Could you check a few things on this model? Use its own coordinates, in mm. Give positions to 0.01 mm unless a question says otherwise; leave off trailing zeros. Loops run counter-clockwise (first coordinate to the right, second up) from the corner with the lowest first, then second, coordinate; pieces in that order, holes last. Notation, with made-up numbers: (24.5, 21) - (72.5, 21) arc R31 ccw to (72.5, 45) - close; hole circle Ø1 at (14.5, 52.25). An arc over 180 degrees is marked (long way). Use CSV: the item, a comma, the result in double quotes.
from build123d import *

# Parameters (mm, degrees)
ESBO_O1_W                         = 130
ESBO_O1_H                         = 55.25
RESSALTO_EXTRUS_O1_DEPTH          = 2.5
ESBO_O2_W                         = 130
ESBO_O2_H                         = 55.25
ESBO_O2_W_2                       = 125
ESBO_O2_H_2                       = 50.25
CORTE_EXTRUS_O1_DEPTH             = 1.25
FUROS_GUIA_COM_3_0MM2_D           = 3
FUROS_GUIA_COM_3_0MM2_CSINK_D     = 3.05
FUROS_GUIA_COM_3_0MM2_CSINK_ANGLE = 90
CUT_EXTRUDE1_DEPTH                = 10
FILETE1_R                         = 2
FURO_COM_FOLGA_DE_M21_D           = 2.4
PADR_O_LINEAR1_COUNT              = 3
PADR_O_LINEAR1_PITCH              = 8
ESPELHAR1_COPY_1_D                = 2.4
ESPELHAR1_COPY_2_D                = 2.4
ESPELHAR2_COPY_1_D                = 2.4
ESPELHAR2_COPY_2_D                = 2.4
ESPELHAR2_COPY_3_D                = 2.4
ESPELHAR2_COPY_4_D                = 2.4
ESPELHAR2_COPY_5_D                = 2.4
FILETE1_OF_ESPELHAR2_R            = 2


with BuildPart() as part:
    # Esboço1 → Ressalto-extrusão1 (new body)
    with BuildSketch(Plane.XY):
        with Locations((1.708397535, 5.726309707)):
            Rectangle(ESBO_O1_W, ESBO_O1_H)
    extrude(amount=RESSALTO_EXTRUS_O1_DEPTH)

    # Esboço2 → Corte-extrusão1 (cut)
    with BuildSketch(Plane.XY.offset(2.5)):
        with Locations((1.708397535, 5.726309707)):
            Rectangle(ESBO_O2_W, ESBO_O2_H)
        with Locations((1.708397535, 5.726309707)):
            Rectangle(ESBO_O2_W_2, ESBO_O2_H_2, mode=Mode.SUBTRACT)
    extrude(amount=-CORTE_EXTRUS_O1_DEPTH, mode=Mode.SUBTRACT)

    # Furos-guia com Ø3.0mm2 (through all)
    with Locations(Plane.XY.offset(2.5)):
        with Locations((-48.791602465, 22.551309707), (-48.791602465, -11.098690293), (52.208397535, -11.098690293), (52.208397535, 22.551309707)):
            CounterSinkHole(FUROS_GUIA_COM_3_0MM2_D / 2, FUROS_GUIA_COM_3_0MM2_CSINK_D / 2, counter_sink_angle=FUROS_GUIA_COM_3_0MM2_CSINK_ANGLE)

    # Sketch1 → Cut-Extrude1 (cut)
    with BuildSketch(Plane.XY.offset(2.5)):
        with BuildLine():
            Line((-39.291602465, -4.773695916), (-15.791602465, -4.773695916))
            Line((-15.791602465, -4.773695916), (-15.791602465, 16.226304084))
            Line((-15.791602465, 16.226304084), (-39.291602465, 16.226304084))
            ThreePointArc((-39.291602465, 16.226304084), (-43.887668713, 13.19109981), (-49.291602465, 12.126304084))
            ThreePointArc((-49.291602465, 12.126304084), (-55.691602465, 5.726304084), (-49.291602465, -0.673695916))
            ThreePointArc((-49.291602465, -0.673695916), (-43.887668713, -1.738491642), (-39.291602465, -4.773695916))
        make_face()
    cut_extrude1 = extrude(amount=-CUT_EXTRUDE1_DEPTH, mode=Mode.SUBTRACT)

    # Filete1
    filete1_edges = [part.edges().sort_by_distance(p)[0] for p in [
        (-39.291602465, -4.773695916, 1.25),
        (-39.291602465, 16.226304084, 1.25),
        (-15.791602465, 16.226304084, 1.25),
        (-15.791602465, -4.773695916, 1.25),
    ]]
    fillet(filete1_edges, radius=FILETE1_R)

    # Furo com folga de M21 (through all)
    with Locations(Plane.XY.offset(2.5)):
        with Locations((37.958397535, -7.773690293)):
            furo_com_folga_de_m21 = Hole(FURO_COM_FOLGA_DE_M21_D / 2)

    # Padrão linear1: Furo com folga de M21 ×3
    with Locations(*[(-i * PADR_O_LINEAR1_PITCH, 0, 0) for i in range(1, PADR_O_LINEAR1_COUNT)]):
        add(furo_com_folga_de_m21, mode=Mode.SUBTRACT)

    # Espelhar1: Furo com folga de M21 across plane
    add(furo_com_folga_de_m21.mirror(Plane(origin=(0, 5.726309707, 0), x_dir=(0, 0, 1), z_dir=(0, -1, 0))), mode=Mode.SUBTRACT)

    # Espelhar1 copy 1 (through all)
    with Locations(Plane(origin=(-8, 11.452619414, 2.5), x_dir=(1, 0, 0), z_dir=(0, 0, 1))):
        with Locations((37.958397535, 7.773690293)):
            Hole(ESPELHAR1_COPY_1_D / 2)

    # Espelhar1 copy 2 (through all)
    with Locations(Plane(origin=(-16, 11.452619414, 2.5), x_dir=(1, 0, 0), z_dir=(0, 0, 1))):
        with Locations((37.958397535, 7.773690293)):
            Hole(ESPELHAR1_COPY_2_D / 2)

    # Espelhar2: Cut-Extrude1, Furo com folga de M21 across plane
    add(cut_extrude1.mirror(Plane(origin=(1.708397535, 0, 0), x_dir=(0, 0, 1), z_dir=(1, 0, 0))), mode=Mode.SUBTRACT)
    add(furo_com_folga_de_m21.mirror(Plane(origin=(1.708397535, 0, 0), x_dir=(0, 0, 1), z_dir=(1, 0, 0))), mode=Mode.SUBTRACT)

    # Espelhar2 copy 1 (through all)
    with Locations(Plane(origin=(11.416795069, 0, 2.5), x_dir=(-1, 0, 0), z_dir=(0, 0, 1))):
        with Locations((37.958397535, 7.773690293)):
            Hole(ESPELHAR2_COPY_1_D / 2)

    # Espelhar2 copy 2 (through all)
    with Locations(Plane(origin=(19.416795069, 0, 2.5), x_dir=(-1, 0, 0), z_dir=(0, 0, 1))):
        with Locations((37.958397535, 7.773690293)):
            Hole(ESPELHAR2_COPY_2_D / 2)

    # Espelhar2 copy 3 (through all)
    with Locations(Plane(origin=(3.416795069, 11.452619414, 2.5), x_dir=(-1, 0, 0), z_dir=(0, 0, 1))):
        with Locations((37.958397535, -7.773690293)):
            Hole(ESPELHAR2_COPY_3_D / 2)

    # Espelhar2 copy 4 (through all)
    with Locations(Plane(origin=(11.416795069, 11.452619414, 2.5), x_dir=(-1, 0, 0), z_dir=(0, 0, 1))):
        with Locations((37.958397535, -7.773690293)):
            Hole(ESPELHAR2_COPY_4_D / 2)

    # Espelhar2 copy 5 (through all)
    with Locations(Plane(origin=(19.416795069, 11.452619414, 2.5), x_dir=(-1, 0, 0), z_dir=(0, 0, 1))):
        with Locations((37.958397535, -7.773690293)):
            Hole(ESPELHAR2_COPY_5_D / 2)

    # Filete1 of Espelhar2
    filete1_of_espelhar2_edges = [part.edges().sort_by_distance(p)[0] for p in [
        (42.708397535, -4.773695916, 1.25),
        (42.708397535, 16.226304084, 1.25),
        (19.208397535, 16.226304084, 1.25),
        (19.208397535, -4.773695916, 1.25),
    ]]
    fillet(filete1_of_espelhar2_edges, radius=FILETE1_OF_ESPELHAR2_R)


solid = part.part
1) We'd pull the mould along Y, two halves only. Please class faces 1 (the cylindrical face through (38.219, -8.945, 1.232)), 2 (the flat face through (1, 6, 0)): +Y half, -Y half, draft (parallel to the pull), parting line (faces both ways), or undercut.
Answer below:
face 1,"undercut"
face 2,"draft"
2) Suppose I cut it at C-C (x = 6). Please give me the cut outline in (y, z), plus the area to 3 significant figures.
Answer below:
outline,"(-21.9, 0) - (33.35, 0) - (33.35, 1.25) - (30.85, 1.25) - (30.85, 2.5) - (-19.4, 2.5) - (-19.4, 1.25) - (-21.9, 1.25) - close"
area,"132 mm2"
3) I need wall thicknesses on line 1 along X through (y, z) = (-3.5, 2.1); line 2 along X through (y, z) = (21.5, 1.3); line 3 along Y through (x, z) = (-31.5, 1.9). Which ranges of each line are inside material? Lowest first, please.
Answer below:
line 1,"x = -60.79 to -40.77, -15.93 to 19.34, 44.19 to 64.21"
line 2,"x = -60.79 to -49.86, -47.72 to 51.14, 53.28 to 64.21"
line 3,"y = -19.4 to -4.77, 16.23 to 30.85"
4) Suppose I cut it at A-A (y = -15). Please give me the cut outline in (x, z), plus the area to 3 significant figures.
Answer below:
outline,"(-63.29, 0) - (66.71, 0) - (66.71, 1.25) - (64.21, 1.25) - (64.21, 2.5) - (-60.79, 2.5) - (-60.79, 1.25) - (-63.29, 1.25) - close"
area,"319 mm2"
5) Suppose I cut it at D-D (y = 3.5). Please give me the cut outline in (x, z).
Answer below:
outline,"(-63.29, 0) - (-55.29, 0) - (-55.29, 2.5) - (-60.79, 2.5) - (-60.79, 1.25) - (-63.29, 1.25) - close; (-15.79, 0) - (19.21, 0) - (19.21, 2.5) - (-15.79, 2.5) - close; (58.71, 0) - (66.71, 0) - (66.71, 1.25) - (64.21, 1.25) - (64.21, 2.5) - (58.71, 2.5) - close"
6) I'm going to push flat-ended pins straight in: P1, Ø1.4, axis at x = 7.5, z = 2, coming from the -Y side; P2, Ø1, axis at y = -3, z = 2, coming from the +X side. Where does each tip first touch, or does it pass through?
Answer below:
P1,"stops at y = -19.4"
P2,"stops at x = 64.21"
7) Suppose I cut it at B-B (x = 46.5). Please give me the cut outline in (y, z), plus the area to 3 significant figures.
Answer below:
outline,"(-21.9, 0) - (-2.1, 0) - (-2.1, 2.5) - (-19.4, 2.5) - (-19.4, 1.25) - (-21.9, 1.25) - close; (13.55, 0) - (33.35, 0) - (33.35, 1.25) - (30.85, 1.25) - (30.85, 2.5) - (13.55, 2.5) - close"
area,"92.8 mm2"
